Verification items for the finished model (mm, model axes). A direction names the side the tool comes from. Round coordinates to 2 decimals unless told otherwise and drop trailing zeros. Write each loop counter-clockwise with the first axis right and the second up, starting at its lowest first coordinate (ties: lowest second). Pieces come first, ordered by that corner, then holes. Notation, with made-up numbers: M 13.25,67.25 L 21.25,67.25 A27 ccw 21.25,88.25 Z; hole C -15.75,10.25 d4. An arc over 180 degrees is marked long. One line per item, written item: value. Start each with the question number.
Item 1: Section check A-A, the plane x = -7.5. Record the cut outline in (y, z).
Item 2: Section check C-C, the plane y = -23.5. Record the cut outline in (x, z).
Item 3: Section check D-D, the plane y = -48. Record the cut outline in (x, z), then the cut area to 3 significant figures.
Item 4: Draft check along Y on faces 5 (the face through (10, -55, -16)), 6 (the face through (17, -47, -3)), 7 (the face through (-12, -40, -17.8)), 8 (the face through (17, -31, -3)). Enter one of: +Y half, -Y half, draft (parallel to the pull), parting line (faces both ways), or undercut.
Item 5: Gauge pin test, flat ends, axial feed: pin 1 (2 mm diameter, centred on x = 13.5, y = -43, fed in from +Z); pin 2 (8 mm diameter, centred on y = -20, z = 2.5, fed in from +X); pin 3 (0.9 mm diameter, centred on x = 22.5, y = -52, fed in from +Z). Record the tip position at first contact, or that the pin passes through.
Item 6: Tool access check on faces 1 (the face through (13.907, -54.494, 0.286)), 2 (the face through (10.9, -40, -2)), 3 (the face through (-23.7, -15, 0)), 4 (the face through (20.9, -27, -13)). Record the directions out of +Z, -Z, +X, -X, +Y, -Y that give a thin tool (end or side, any length) a straight path to the whole face; none if there is none.
Item 7: Thickness scan on probe 1 along Y at (x, z) = (15.5, 0); probe 2 along Y at (x, z) = (-14, -10.5); probe 3 along Y at (x, z) = (-22, 20.5). Record the ranges inside material, lowest first. Write a range as from..to.
Item 8: Section check B-B, the plane z = -9. Record the cut outline in (x, y), then the cut area to 3 significant figures.
from build123d import *

# Parameters (mm, degrees)
F1_DEPTH  = 55
F3_DEPTH  = 30
F4_R      = 3
F5_DEPTH  = 25
F6_R      = 12.5
F7_DEPTH  = 25
F8_R      = 15
F9_DEPTH  = 38
F10_R     = 15
F11_DEPTH = 8
F12_R     = 6.5
F13_DEPTH = 17
F14_R     = 10


with BuildPart() as f1:
    # F0 (on Front) → F1 (new body)
    with BuildSketch(Plane.XZ):
        with BuildLine():
            Line((-23.699999, 23.799999), (-23.699999, 23.558845))
            Line((-23.699999, 23.558845), (-24.369059, 22.399999))
            Line((-24.369059, 22.399999), (-23.699999, 21.241153))
            Line((-23.699999, 21.241153), (-23.699999, -21.000001))
            ThreePointArc((-23.699999, -21.000001), (-22.001218, -25.10122), (-17.899999, -26.8))
            Line((-17.899999, -26.8), (15.100001, -26.8))
            ThreePointArc((15.100001, -26.8), (19.20122, -25.10122), (20.9, -21.000001))
            Line((20.9, -21.000001), (20.9, -4.000001))
            ThreePointArc((20.9, -4.000001), (21.251472, -3.151472), (22.100001, -2.8))
            Line((22.100001, -2.8), (22.9, -2.8))
            Line((22.9, -2.8), (22.9, 2.799999))
            Line((22.9, 2.799999), (22.100001, 2.799999))
            ThreePointArc((22.100001, 2.799999), (21.251472, 3.151471), (20.9, 3.999999))
            Line((20.9, 3.999999), (20.9, 11.499999))
            ThreePointArc((20.9, 11.499999), (21.397919, 12.702081), (22.600001, 13.2))
            Line((22.600001, 13.2), (23.100001, 13.2))
            ThreePointArc((23.100001, 13.2), (23.665686, 13.434314), (23.9, 13.999999))
            Line((23.9, 13.999999), (23.9, 21.241153))
            Line((23.9, 21.241153), (24.56906, 22.399999))
            Line((24.56906, 22.399999), (23.9, 23.558845))
            Line((23.9, 23.558845), (23.9, 23.799999))
            Line((23.9, 23.799999), (-23.699999, 23.799999))
        make_face()
    extrude(amount=F1_DEPTH)

    # F2 (on face) → F3 (cut)
    with BuildSketch(Plane.XZ.offset(55)):
        with BuildLine():
            Line((15.9, 11.457851), (26.682628, 11.457851))
            Line((26.682628, 11.457851), (26.682628, 26.709846))
            Line((26.682628, 26.709846), (-26.825872, 26.709846))
            Line((-26.825872, 26.709846), (-26.825872, -17.8))
            Line((-26.825872, -17.8), (5.9, -17.8))
            Line((5.9, -17.8), (10.9, -17.8))
            Line((10.9, -17.8), (10.9, -11.8))
            Line((10.9, -11.8), (10.9, 6.457851))
            ThreePointArc((10.9, 6.457851), (12.364466, 9.993385), (15.9, 11.457851))
        make_face()
    extrude(amount=-F3_DEPTH, mode=Mode.SUBTRACT)

    # F4 (on face) → F5 (cut)
    with BuildSketch(Plane.YZ.offset(22.9)):
        with Locations((-48, -1e-06)):
            Circle(F4_R)
        with Locations((-32, -1e-06)):
            Circle(F4_R)
    extrude(amount=-F5_DEPTH, mode=Mode.SUBTRACT)

    # F6 (on face) → F7 (cut, through all)
    with BuildSketch(Plane(origin=(0, 0, 0), x_dir=(-1, 0, 0), z_dir=(0, 1, 0))):
        with Locations((5.799999, -0.9)):
            Circle(F6_R)
    extrude(amount=-F7_DEPTH, mode=Mode.SUBTRACT)

    # F8 (on face) → F9 (cut)
    with BuildSketch(Plane.XZ.offset(55)):
        with Locations((-5.799999, -0.9)):
            Circle(F8_R)
    extrude(amount=-F9_DEPTH, mode=Mode.SUBTRACT)

    # F10 (on face) → F11 (cut)
    with BuildSketch(Plane(origin=(0, 0, 0), x_dir=(-1, 0, 0), z_dir=(0, 1, 0))):
        with Locations((5.799999, -0.9)):
            Circle(F10_R)
    extrude(amount=-F11_DEPTH, mode=Mode.SUBTRACT)

    # F12 (on Right) → F13 (cut)
    with BuildSketch(Plane.YZ):
        with Locations((-32, 0)):
            Circle(F12_R)
        with Locations((-48, 0)):
            Circle(F12_R)
    extrude(amount=F13_DEPTH, mode=Mode.SUBTRACT)

    # F14
    f14_edges = [f1.edges().sort_by_distance(p)[0] for p in [
        (10.9, -40, -17.8),
    ]]
    fillet(f14_edges, radius=F14_R)


solid = f1.part
Response values:
1. outline: M -55,-26.8 L 0,-26.8 L 0,-15.8 L -8,-15.8 L -8,-13.28 L -17,-13.28 L -17,-15.8 L -25,-15.8 L -25,-17.8 L -55,-17.8 Z; M -25,14 L -17,14 L -17,11.48 L -8,11.48 L -8,14 L 0,14 L 0,23.8 L -25,23.8 Z
2. outline: M -24.37,22.4 L -23.7,21.24 L -23.7,-21 A5.8 ccw -17.9,-26.8 L 15.1,-26.8 A5.8 ccw 20.9,-21 L 20.9,-4 A1.2 cw 22.1,-2.8 L 22.9,-2.8 L 22.9,2.8 L 22.1,2.8 A1.2 cw 20.9,4 L 20.9,11.5 A1.7 cw 22.6,13.2 L 23.1,13.2 A0.8 ccw 23.9,14 L 23.9,21.24 L 24.57,22.4 L 23.9,23.56 L 23.9,23.8 L -23.7,23.8 L -23.7,23.56 Z; hole C -5.8,-0.9 d30
3. outline: M -23.7,-21 A5.8 ccw -17.9,-26.8 L 15.1,-26.8 A5.8 ccw 20.9,-21 L 20.9,-4 A1.2 cw 21.44,-3 L 17,-3 L 17,-6.5 L 10.9,-6.5 L 10.9,-7.8 A10 cw 0.9,-17.8 L -23.7,-17.8 Z; M 10.9,6.5 L 17,6.5 L 17,3 L 21.44,3 A1.2 cw 20.9,4 L 20.9,11.46 L 15.9,11.46 A5 ccw Z
3. area: 593 mm2
4. face 5: -Y half
4. face 6: undercut
4. face 7: draft
4. face 8: undercut
5. pin 1: stops at z = 11.26
5. pin 2: stops at x = 22.9
5. pin 3: stops at z = 2.8
6. face 1: -X
6. face 2: +Z, -X, -Y
6. face 3: -Z, -X, +Y, -Y
6. face 4: -Z, +X, +Y, -Y
7. probe 1: y = -55..-54.5, -41.5..-38.5, -25.5..0
7. probe 2: y = -17..-8
7. probe 3: y = -25..0
8. outline: M -23.7,-25 L -18.42,-25 L -18.42,-17 L -15.32,-17 L -15.32,-8 L -18.42,-8 L -18.42,0 L -23.7,0 Z; M 3.72,-17 L 6.82,-17 L 6.82,-25 L 10.83,-25 L 10.83,-55 L 20.9,-55 L 20.9,0 L 6.82,0 L 6.82,-8 L 3.72,-8 Z
8. area: 842 mm2
